from build123d import *

# Parameters (mm, degrees)
F0_W     = 50.8
F0_H     = 63.5
F1_DEPTH = 53.975
F3_DEPTH = 50.801
F4_R     = 7.9375
F5_DEPTH = 107.951


with BuildPart() as f1:
    # F0 (on Top) → F1 (new body, symmetric)
    with BuildSketch(Plane.XY):
        with Locations((0, 31.75)):
            Rectangle(F0_W, F0_H)
        with BuildLine():
            Line((25.4, 0), (-25.4, 0))
            ThreePointArc((-25.4, 0), (0, -25.4), (25.4, 0))
        make_face()
    extrude(amount=F1_DEPTH, both=True)

    # F2 (on face) → F3 (cut, through all)
    with BuildSketch(Plane.YZ.offset(25.4)):
        Polygon((0, 0), (0, 47.625), (-25.4, 47.625), (-25.4, -47.625), (0, -47.625), align=None)
        Polygon((38.1, -47.625), (38.1, 47.625), (0, 47.625), (0, 0), (0, -47.625), align=None)
    extrude(amount=-F3_DEPTH, mode=Mode.SUBTRACT)

    # F4 (on face) → F5 (cut, through all)
    with BuildSketch(Plane.XY.offset(53.975)):
        Circle(F4_R)
    extrude(amount=-F5_DEPTH, mode=Mode.SUBTRACT)


solid = f1.part
Model file for the job. Use its own axes, mm. A direction names the side the tool comes from. Coordinates: 2 decimals unless noted, no trailing zeros. Loops run counter-clockwise (first coordinate to the right, second up) from the corner with the lowest first, then second, coordinate; pieces in that order, holes last. Notation, with made-up numbers: (82.25, -1.75) -> (92.25, -1.75) arc R4 cw to (92.25, 5.25) -> close; hole circle Ø1 at (58, -12). An arc over 180 degrees is marked (long way). Use one line per item in the form item = value. Start each with the question number.
(1) Cut at A-A on x = 0. Give the cut face in (y, z) (1 decimal).
(2) Cut at C-C on y = 4. Give the cut face in (x, z) (3 decimals), and give its area (3 significant figures).
(3) Tool access for faces 4 (the flat face through (0, 14, 47.625)), 5 (the flat face through (0, 63.5, 1)): list every direction of +Z, -Z, +X, -X, +Y, -Y with a clear straight run to the whole face (end or side of a thin tool).
(4) Cut at B-B on y = 17. Give the cut face in (x, z) (3 decimals), and give its area (3 significant figures).
(5) Probe probe 1 along Z at (x, y) = (12.5, -10) (3 decimals); probe 2 along Y at (x, z) = (0, 51); probe 3 along Y at (x, z) = (5, -46.5). List the from-to ranges inside material, lowest first. Write a range as from..to.
(6) Pull direction X, two halves, no side cores. Call faces 1 (the cylindrical face through (-1.72, -7.75, -50.76)), 2 (the flat face through (0, 38.1, -1)), 3 (the cylindrical face through (-0.559, -25.394, 50.844)): pulls with the +X half, pulls with the -X half, needs draft (parallel to the pull), parting line crosses it, or undercut.
(7) Cut at D-D on x = 13. Give the cut face in (y, z) (3 decimals).
(8) Flat gauge pin, fed straight in: pin 1 (20.5 mm diameter, centred on x = 0, y = 0, fed in from -Z) (3 decimals). Where does the tip first touch, or does it go through?
Values:
q1.outline = (-25.4, -54) -> (-7.9, -54) -> (-7.9, -47.6) -> (-25.4, -47.6) -> close; (-25.4, 47.6) -> (-7.9, 47.6) -> (-7.9, 54) -> (-25.4, 54) -> close; (7.9, -54) -> (63.5, -54) -> (63.5, 54) -> (7.9, 54) -> (7.9, 47.6) -> (38.1, 47.6) -> (38.1, -47.6) -> (7.9, -47.6) -> close
q2.outline = (-25.4, -53.975) -> (-6.856, -53.975) -> (-6.856, -47.625) -> (-25.4, -47.625) -> close; (-25.4, 47.625) -> (-6.856, 47.625) -> (-6.856, 53.975) -> (-25.4, 53.975) -> close; (6.856, -53.975) -> (25.4, -53.975) -> (25.4, -47.625) -> (6.856, -47.625) -> close; (6.856, 47.625) -> (25.4, 47.625) -> (25.4, 53.975) -> (6.856, 53.975) -> close
q2.area = 471 mm2
q3.face_4 = +X, -X, -Y
q3.face_5 = +Z, -Z, +X, -X, +Y
q4.outline = (-25.4, -53.975) -> (25.4, -53.975) -> (25.4, -47.625) -> (-25.4, -47.625) -> close; (-25.4, 47.625) -> (25.4, 47.625) -> (25.4, 53.975) -> (-25.4, 53.975) -> close
q4.area = 645 mm2
q5.probe_1 = -53.975..-47.625, 47.625..53.975
q5.probe_2 = -25.4..-7.94, 7.94..63.5
q5.probe_3 = 38.1..63.5
q6.face_1 = undercut
q6.face_2 = needs draft
q6.face_3 = parting line crosses it
q7.outline = (-21.821, -53.975) -> (63.5, -53.975) -> (63.5, 53.975) -> (-21.821, 53.975) -> (-21.821, 47.625) -> (38.1, 47.625) -> (38.1, -47.625) -> (-21.821, -47.625) -> close
q8.pin_1 = -53.975
